Check sheet for the modelled part. Datum: model origin and axes. Units: mm. A direction names the side the tool comes from. Coordinates: 2 decimals unless noted, no trailing zeros. Loops run counter-clockwise (first coordinate to the right, second up) from the corner with the lowest first, then second, coordinate; pieces in that order, holes last.
from build123d import *

# Parameters (mm, degrees)
F1_DEPTH = 1.5
F2_W     = 4.974715
F2_H     = 3.17829
F3_DEPTH = 2.5


with BuildPart() as f1:
    # F0 (on Front) → F1 (new body, symmetric)
    with BuildSketch(Plane.XZ):
        Polygon((-48.918031, 0), (-43.666944, 0), (-17.964249, 0), (-17.964249, 2.625544), (-48.918031, 2.625544), align=None)
    extrude(amount=F1_DEPTH, both=True)

    # F2 (on Front) → F3 (join, symmetric)
    with BuildSketch(Plane.XZ):
        with Locations((-43.114196, -1.589145)):
            Rectangle(F2_W, F2_H)
    extrude(amount=F3_DEPTH, both=True)


solid = f1.part
(1) Gauge pin test, flat ends, axial feed: P1, Ø2.5, axis at x = -47, y = 0, coming from the -Z side; P2, Ø1.3, axis at x = -39, z = 1.5, coming from the -Y side; P3, Ø1.3, axis at x = -35.5, z = 2, coming from the +Y side. Record the tip position at first contact, or that the pin passes through.
(2) Set-up check for faces 1 (the face through (-43, 2, 0)), 2 (the face through (-40.627, 0, -2)), 3 (the face through (-45.602, 0, -2)): record each of +Z, -Z, +X, -X, +Y, -Y from which the full face is reachable in a straight line by a thin tool's end or side.
(3) Section check D-D, the plane z = -1.65. Enter the section's corners in (x, y), plus the area to 3 significant figures.
(4) Scan lines: line 1 along Y through (x, z) = (-28, 1.45); line 2 along X through (y, z) = (-0.6, -1.6); line 3 along Z through (x, y) = (-22, 0.5). Record each from-to range of solid material in increasing order.
(5) Section check B-B, the plane y = -0.45. Enter the section's corners in (x, z).
(6) Section check C-C, the plane z = 1.5. Enter the section's corners in (x, y), plus the area to 3 significant figures.
(7) Section check A-A, the plane x = -42. Enter the section's corners in (y, z).
Determined:
1. P1: stops at z = 0
1. P2: stops at y = -1.5
1. P3: stops at y = 1.5
2. face 1: +Z, +X, -X, +Y
2. face 2: -Z, +X, +Y, -Y
2. face 3: -Z, -X, +Y, -Y
3. outline: (-45.6, -2.5) - (-40.63, -2.5) - (-40.63, 2.5) - (-45.6, 2.5) - close
3. area: 24.9 mm2
4. line 1: y = -1.5 to 1.5
4. line 2: x = -45.6 to -40.63
4. line 3: z = 0 to 2.63
5. outline: (-48.92, 0) - (-45.6, 0) - (-45.6, -3.18) - (-40.63, -3.18) - (-40.63, 0) - (-17.96, 0) - (-17.96, 2.63) - (-48.92, 2.63) - close
6. outline: (-48.92, -1.5) - (-17.96, -1.5) - (-17.96, 1.5) - (-48.92, 1.5) - close
6. area: 92.9 mm2
7. outline: (-2.5, -3.18) - (2.5, -3.18) - (2.5, 0) - (1.5, 0) - (1.5, 2.63) - (-1.5, 2.63) - (-1.5, 0) - (-2.5, 0) - close
